from build123d import *

# Parameters (mm, degrees)
ESBO_O1_W                = 10
ESBO_O1_H                = 3
RESSALTO_EXTRUS_O1_DEPTH = 5
ESBO_O4_W                = 1
ESBO_O4_H                = 1.5
RESSALTO_EXTRUS_O2_DEPTH = 1
ESBO_O8_W                = 2
ESBO_O8_H                = 1.5
CORTE_EXTRUS_O2_DEPTH    = 0.5
CORTE_EXTRUS_O5_DEPTH    = 0.1
CORTE_EXTRUS_O6_DEPTH    = 0.5
ESBO_O11_R               = 0.4
RESSALTO_EXTRUS_O4_DEPTH = 3
ESBO_O19_W               = 3
ESBO_O19_H               = 2
CORTE_EXTRUS_O9_DEPTH    = 0.5
ESBO_O21_W               = 2.995544047
ESBO_O21_H               = 1
CORTE_EXTRUS_O10_DEPTH   = 0.3


with BuildPart() as part:
    # Esboço1 → Ressalto-extrusão1 (new body)
    with BuildSketch(Plane(origin=(0, 0, 0), x_dir=(1, 0, 0), z_dir=(0, 1, 0))):
        with Locations((5, 1.5)):
            Rectangle(ESBO_O1_W, ESBO_O1_H)
    extrude(amount=RESSALTO_EXTRUS_O1_DEPTH)

    # Esboço4 → Ressalto-extrusão2 (add)
    with BuildSketch(Plane(origin=(0, 5, 0), x_dir=(1, 0, 0), z_dir=(0, 1, 0))):
        with Locations((3.5, 1.25)):
            Rectangle(ESBO_O4_W, ESBO_O4_H)
    extrude(amount=RESSALTO_EXTRUS_O2_DEPTH)

    # Esboço8 → Corte-extrusão2 (cut)
    with BuildSketch(Plane(origin=(0, 5, 0), x_dir=(1, 0, 0), z_dir=(0, 1, 0))):
        with Locations((5, 1.25)):
            Rectangle(ESBO_O8_W, ESBO_O8_H)
    extrude(amount=-CORTE_EXTRUS_O2_DEPTH, mode=Mode.SUBTRACT)

    # Esboço9 → Corte-extrusão5 (cut)
    with BuildSketch(Plane(origin=(0, 5, 0), x_dir=(1, 0, 0), z_dir=(0, 1, 0))):
        with BuildLine():
            add(Edge.make_bspline(
                [(7.717025162, 2.685064935), (7.768275073, 2.684653139), (7.867968532, 2.683852096), (8.012830606, 2.675522502), (8.148601104, 2.662599241), (8.275087284, 2.644432886), (8.392605867, 2.621489185), (8.500848932, 2.592511147), (8.600323781, 2.558959581), (8.689910066, 2.519182744), (8.770052693, 2.476635016), (8.839594359, 2.430662628), (8.899331263, 2.382896177), (8.947218272, 2.331040045), (8.986118217, 2.27759415), (9.012308422, 2.220411921), (9.029958288, 2.161052106), (9.031626399, 2.120222692), (9.032467532, 2.09963474)],
                knots=[0, 0, 0, 0, 0.000153734, 0.000299051, 0.000435142, 0.000562774, 0.000682263, 0.000794121, 0.000898722, 0.000996847, 0.001087864, 0.001170597, 0.00124666, 0.001316656, 0.001381822, 0.001444006, 0.001504562, 0.001566156, 0.001566156, 0.001566156, 0.001566156], degree=3))
            add(Edge.make_bspline(
                [(9.032467532, 2.09963474), (9.031952466, 2.086243406), (9.03092816, 2.059612265), (9.023519116, 2.020284156), (9.011816828, 1.98174038), (8.994996923, 1.944322939), (8.973326429, 1.907779642), (8.946647613, 1.872377676), (8.91588358, 1.837308554), (8.879929464, 1.803879089), (8.84003574, 1.771271209), (8.79508583, 1.741089795), (8.746201299, 1.712010826), (8.693008442, 1.684722634), (8.635338402, 1.659358364), (8.573479622, 1.635698049), (8.507410398, 1.613183974), (8.437075438, 1.593196089), (8.363020356, 1.57481891), (8.285320249, 1.559134103), (8.204039884, 1.546195816), (8.119518678, 1.534740096), (8.031299129, 1.526956469), (7.939792349, 1.520962638), (7.844740014, 1.516511464), (7.78027454, 1.516327433), (7.747463474, 1.516233766)],
                knots=[0, 0, 0, 0, 4.0157e-05, 7.986e-05, 0.000119657, 0.000160761, 0.00020261, 0.000246848, 0.000293569, 0.000342376, 0.000393954, 0.000447987, 0.000504626, 0.000564524, 0.000627211, 0.000693536, 0.000763161, 0.000836538, 0.000912823, 0.000992017, 0.001074251, 0.001159703, 0.001247841, 0.001339865, 0.001434818, 0.00153324, 0.00153324, 0.00153324, 0.00153324], degree=3))
            add(Edge.make_bspline(
                [(7.747463474, 1.516233766), (7.702642019, 1.51673791), (7.614970919, 1.517724018), (7.486687775, 1.524909023), (7.364657949, 1.536494006), (7.248954096, 1.552416836), (7.139735974, 1.573715014), (7.036976444, 1.599695769), (6.940209946, 1.629432703), (6.87929448, 1.654605061), (6.849533279, 1.666903409)],
                knots=[0, 0, 0, 0, 0.00013446, 0.000263004, 0.000385315, 0.000502115, 0.000613247, 0.000718938, 0.000820018, 0.000916578, 0.000916578, 0.000916578, 0.000916578], degree=3))
            add(Edge.make_bspline(
                [(6.849533279, 1.666903409), (6.819495721, 1.680737693), (6.762099909, 1.707172265), (6.684107261, 1.753561383), (6.617281662, 1.802485084), (6.562765507, 1.855474257), (6.520316361, 1.9119252), (6.489575578, 1.97162645), (6.471096623, 2.035136967), (6.468725659, 2.078717419), (6.467532468, 2.100649351)],
                knots=[0, 0, 0, 0, 9.9153e-05, 0.000189462, 0.000271747, 0.000347082, 0.000416684, 0.000482706, 0.000547582, 0.000613307, 0.000613307, 0.000613307, 0.000613307], degree=3))
            add(Edge.make_bspline(
                [(6.467532468, 2.100649351), (6.468673515, 2.122760058), (6.470934698, 2.166576254), (6.490149361, 2.23047144), (6.521930555, 2.290377771), (6.565195504, 2.347502443), (6.621476513, 2.400294414), (6.689828213, 2.449371296), (6.769790362, 2.49578785), (6.828783463, 2.521791334), (6.859679383, 2.535409903)],
                knots=[0, 0, 0, 0, 6.623e-05, 0.000131246, 0.000198184, 0.000268801, 0.000345229, 0.000428739, 0.000520798, 0.000622027, 0.000622027, 0.000622027, 0.000622027], degree=3))
            add(Edge.make_bspline(
                [(6.859679383, 2.535409903), (6.889983671, 2.547446904), (6.951310735, 2.571806293), (7.047289586, 2.602023308), (7.147652813, 2.628051521), (7.252801276, 2.648342721), (7.36221225, 2.665485653), (7.476356384, 2.676921818), (7.595195642, 2.68340278), (7.675925466, 2.6845042), (7.717025162, 2.685064935)],
                knots=[0, 0, 0, 0, 9.7794e-05, 0.000197907, 0.000301632, 0.000408684, 0.000519032, 0.000633771, 0.000752663, 0.000875964, 0.000875964, 0.000875964, 0.000875964], degree=3))
        make_face()
        with BuildLine():
            add(Edge.make_bspline(
                [(7.712966721, 2.522727273), (7.676265876, 2.522308225), (7.605018602, 2.52149473), (7.50124071, 2.516066621), (7.403787401, 2.506272361), (7.312351828, 2.493718156), (7.227668706, 2.475551712), (7.149030594, 2.455141256), (7.076719376, 2.430343071), (7.011040089, 2.401515886), (6.952378669, 2.370275717), (6.901011675, 2.337541762), (6.858096688, 2.302123084), (6.822086823, 2.265855819), (6.794084242, 2.227459146), (6.774410061, 2.1871143), (6.762168952, 2.14498675), (6.760550491, 2.116116802), (6.75974026, 2.101663961)],
                knots=[0, 0, 0, 0, 0.000110104, 0.000213745, 0.000311623, 0.000403886, 0.000490446, 0.000571292, 0.000647498, 0.000719509, 0.000786234, 0.00084674, 0.000901887, 0.00095283, 0.000999714, 0.00104373, 0.001086934, 0.001130246, 0.001130246, 0.001130246, 0.001130246], degree=3))
            add(Edge.make_bspline(
                [(6.75974026, 2.101663961), (6.760546361, 2.08687607), (6.762147128, 2.057510041), (6.774313031, 2.014588099), (6.794620069, 1.973819375), (6.82312444, 1.935125343), (6.858951297, 1.897980531), (6.902606815, 1.862790076), (6.954424216, 1.830037922), (7.013593655, 1.798559592), (7.080701403, 1.770420052), (7.15507718, 1.745439683), (7.237089191, 1.7250245), (7.326311037, 1.707753487), (7.423058943, 1.694892365), (7.527126513, 1.685211994), (7.638673744, 1.679804459), (7.715497711, 1.678990654), (7.755073052, 1.678571429)],
                knots=[0, 0, 0, 0, 4.4322e-05, 8.8015e-05, 0.00013271, 0.000180302, 0.00023161, 0.00028715, 0.000348081, 0.000415255, 0.000487996, 0.000566123, 0.000650406, 0.000741342, 0.000838628, 0.000943072, 0.001054818, 0.001173545, 0.001173545, 0.001173545, 0.001173545], degree=3))
            add(Edge.make_bspline(
                [(7.755073052, 1.678571429), (7.806337615, 1.67933264), (7.906298407, 1.680816928), (8.051928946, 1.692847075), (8.189578018, 1.711140794), (8.277380562, 1.731189916), (8.320211039, 1.740969968)],
                knots=[0, 0, 0, 0, 0.000153767, 0.00029983, 0.000438153, 0.000569888, 0.000569888, 0.000569888, 0.000569888], degree=3))
            add(Edge.make_bspline(
                [(8.320211039, 1.740969968), (8.350692489, 1.749465777), (8.409390915, 1.765826239), (8.490866203, 1.799714474), (8.563441842, 1.83845794), (8.625079395, 1.883949286), (8.675708543, 1.933016459), (8.713082539, 1.985414753), (8.736039938, 2.041202632), (8.738865882, 2.07965435), (8.74025974, 2.09862013)],
                knots=[0, 0, 0, 0, 9.485e-05, 0.000182653, 0.000264154, 0.000341064, 0.000411733, 0.000474779, 0.000533093, 0.00058985, 0.00058985, 0.00058985, 0.00058985], degree=3))
            add(Edge.make_bspline(
                [(8.74025974, 2.09862013), (8.739452698, 2.113743816), (8.737850374, 2.143770825), (8.725711477, 2.187701113), (8.705482151, 2.229237127), (8.67758473, 2.268647264), (8.642026485, 2.305993002), (8.598385597, 2.341015015), (8.546814492, 2.373728066), (8.487776446, 2.404835686), (8.420389396, 2.432702421), (8.344485848, 2.456804565), (8.260267259, 2.477516021), (8.167366142, 2.493969498), (8.065977549, 2.507157629), (7.955920014, 2.515874448), (7.837316624, 2.521580425), (7.755418511, 2.522335751), (7.712966721, 2.522727273)],
                knots=[0, 0, 0, 0, 4.5332e-05, 9.0004e-05, 0.000135611, 0.000183322, 0.00023428, 0.00028982, 0.000350751, 0.000417239, 0.000489784, 0.000569198, 0.000655941, 0.000749776, 0.000852091, 0.000962554, 0.001080888, 0.001208238, 0.001208238, 0.001208238, 0.001208238], degree=3))
        make_face(mode=Mode.SUBTRACT)
        Polygon((6.5, 1.321428571), (9, 1.321428571), (9, 1.148944805), (7.035714286, 0.50974026), (9, 0.50974026), (9, 0.347402597), (6.5, 0.347402597), (6.5, 0.520900974), (8.461241883, 1.159090909), (6.5, 1.159090909), align=None)
    extrude(amount=-CORTE_EXTRUS_O5_DEPTH, mode=Mode.SUBTRACT)

    # Esboço10 → Corte-extrusão6 (cut)
    with BuildSketch(Plane(origin=(0, 5, 0), x_dir=(1, 0, 0), z_dir=(0, 1, 0))):
        Polygon((2.5, 1.504407051), (2.5, 1.051282051), (0.5, 1.051282051), (0.5, 1.282051282), (2.294871795, 1.282051282), (2.294871795, 1.641025641), align=None)
    extrude(amount=-CORTE_EXTRUS_O6_DEPTH, mode=Mode.SUBTRACT)

    # Esboço11 → Ressalto-extrusão4 (add)
    with BuildSketch(Plane.XZ):
        with Locations((1, -1.5)):
            Circle(ESBO_O11_R)
        with Locations((9, -1.5)):
            Circle(ESBO_O11_R)
    extrude(amount=RESSALTO_EXTRUS_O4_DEPTH)

    # Esboço19 → Corte-extrusão9 (cut)
    with BuildSketch(Plane(origin=(0, 0, -3), x_dir=(-1, 0, 0), z_dir=(0, 0, -1))):
        with Locations((-4.5, 4)):
            Rectangle(ESBO_O19_W, ESBO_O19_H)
    extrude(amount=-CORTE_EXTRUS_O9_DEPTH, mode=Mode.SUBTRACT)

    # Esboço21 → Corte-extrusão10 (cut)
    with BuildSketch(Plane(origin=(0, 0, -3), x_dir=(-1, 0, 0), z_dir=(0, 0, -1))):
        with Locations((-4.502227977, 2.5)):
            Rectangle(ESBO_O21_W, ESBO_O21_H)
    extrude(amount=-CORTE_EXTRUS_O10_DEPTH, mode=Mode.SUBTRACT)


solid = part.part
Design review of the part built by this model. Coordinates are the model's own, in mm. A direction names the side the tool comes from. Coordinates: 2 decimals unless noted, no trailing zeros. Write each loop counter-clockwise with the first axis right and the second up, starting at its lowest first coordinate (ties: lowest second). Pieces come first, ordered by that corner, then holes. Notation, with made-up numbers: (2, 67) - (56, 67) arc R11 ccw to (56, 75) - close; hole circle Ø6 at (46, -20). An arc over 180 degrees is marked (long way). One line per item, written item: value.
1) For faces 1 (the face through (5, 4.5, -1)), 2 (the face through (8.6, -1.5, -1.5)), 3 (the face through (4.5, 2.5, -2.7)), 4 (the face through (8, 5, -2)), list the 3-axis set-ups (+Z, -Z, +X, -X, +Y, -Y) from which the entire face can be reached by the end or side of a thin tool; tool diameter is ignored.
Answer sheet:
face 1: +Y
face 2: -Y
face 3: -Z, +Y
face 4: +Z, -Z, +X, +Y
2) Add section A-A (x = 1). State the section outline as (y, z) points.
Answer sheet:
outline: (-3, -1.9) - (0, -1.9) - (0, -3) - (5, -3) - (5, -1.28) - (4.5, -1.28) - (4.5, -1.05) - (5, -1.05) - (5, 0) - (0, 0) - (0, -1.1) - (-3, -1.1) - close
3) Add section B-B (y = -1.5). State the section outline as (x, z) points.
Answer sheet:
outline: circle Ø0.8 at (1, -1.5); circle Ø0.8 at (9, -1.5)
4) Mouldability with a two-part tool opening along X and no side actions: class faces 5 (the face through (4.9, 5, -2.2)), 6 (the face through (10, 2, -1)), 7 (the face through (5, 4, -2.5)) as +X half, -X half, draft (parallel to the pull), parting line (faces both ways), or undercut.
Answer sheet:
face 5: draft
face 6: +X half
face 7: undercut
5) Add section C-C (y = 5.25). State the section outline as (x, z) points, plus the area to 3 significant figures.
Answer sheet:
outline: (3, -2) - (4, -2) - (4, -0.5) - (3, -0.5) - close
area: 1.50 mm2
6) Insertion check: pin 1 (1.6 mm diameter, centred on x = 4.5, y = 3.5, fed in from -Z); pin 2 (0.8 mm diameter, centred on y = 5.5, z = -1, fed in from +X); pin 3 (0.8 mm diameter, centred on x = 3.5, y = 5.5, fed in from +Z). Each pin has a flat end and moves straight along its axis. Give the tip position at first contact, or say it passes through.
Answer sheet:
pin 1: stops at z = -2.7
pin 2: stops at x = 4
pin 3: stops at z = -0.5
7) Add section D-D (z = -0.7). State the section outline as (x, y) points.
Answer sheet:
outline: (0, 0) - (10, 0) - (10, 5) - (7.62, 5) - (7.62, 4.9) - (7.05, 4.9) - (7.05, 5) - (6, 5) - (6, 4.5) - (4, 4.5) - (4, 6) - (3, 6) - (3, 5) - (0, 5) - close
